```python
from build123d import *

# Parameters (mm, degrees)
BOSS_EXTRUDE1_DEPTH = 914.4
SKETCH2_R           = 1.5875
CUT_EXTRUDE2_DEPTH  = 2.794
SKETCH4_R           = 1.5875
SKETCH4_R_2         = 3.175
CUT_EXTRUDE3_DEPTH  = 8.89
SKETCH10_W          = 19.05
SKETCH10_H          = 914.4
CUT_EXTRUDE4_DEPTH  = 915.79678891
CUT_EXTRUDE5_REACH  = 916.797
SKETCH11_R          = 3.175


with BuildPart() as part:
    # Sketch1 → Boss-Extrude1 (new body)
    with BuildSketch(Plane.XY):
        Polygon((0, 0), (0, 19.05), (1.5875, 19.05), (1.5875, 1.5875), (19.05, 1.5875), (19.05, 0), align=None)
    boss_extrude1 = extrude(amount=-BOSS_EXTRUDE1_DEPTH)

    # Sketch2 → Cut-Extrude2 (cut)
    with BuildSketch(Plane(origin=(0, 1.5875, 0), x_dir=(1, 0, 0), z_dir=(0, 1, 0))):
        with Locations(Location((9.525, 9.525, 0), (0, 0, 270))):
            Circle(SKETCH2_R)
        with Locations(Location((9.525, 904.875, 0), (0, 0, 270))):
            Circle(SKETCH2_R)
    cut_extrude2 = extrude(amount=-CUT_EXTRUDE2_DEPTH, mode=Mode.SUBTRACT)

    # Sketch4 → Cut-Extrude3 (cut)
    with BuildSketch(Plane(origin=(1.5875, 0, 0), x_dir=(0, 0, -1), z_dir=(1, 0, 0))):
        with Locations((9.525, 9.525)):
            Circle(SKETCH4_R)
        with Locations((904.875, 9.525)):
            Circle(SKETCH4_R)
        with Locations((254, 9.525)):
            Circle(SKETCH4_R_2)
        with Locations((285.75, 9.525)):
            Circle(SKETCH4_R_2)
        with Locations((317.5, 9.525)):
            Circle(SKETCH4_R_2)
        with Locations((349.25, 9.525)):
            Circle(SKETCH4_R_2)
        with Locations((469.9, 9.525)):
            Circle(SKETCH4_R_2)
        with Locations((406.4, 9.525)):
            Circle(SKETCH4_R_2)
        with Locations((438.15, 9.525)):
            Circle(SKETCH4_R_2)
        with Locations((374.65, 9.525)):
            Circle(SKETCH4_R_2)
    cut_extrude3 = extrude(amount=-CUT_EXTRUDE3_DEPTH, mode=Mode.SUBTRACT)

    # Mirror1: Boss-Extrude1, Cut-Extrude2, Cut-Extrude3 across plane
    add(boss_extrude1.mirror(Plane(origin=(0, 19.05, -914.4), x_dir=(0, 0, 1), z_dir=(0, 1, 0))))
    add(cut_extrude2.mirror(Plane(origin=(0, 19.05, -914.4), x_dir=(0, 0, 1), z_dir=(0, 1, 0))), mode=Mode.SUBTRACT)
    add(cut_extrude3.mirror(Plane(origin=(0, 19.05, -914.4), x_dir=(0, 0, 1), z_dir=(0, 1, 0))), mode=Mode.SUBTRACT)

    # Sketch10 → Cut-Extrude4 (cut, through all)
    with BuildSketch(Plane(origin=(0, 19.05, 0), x_dir=(-1, 0, 0), z_dir=(0, -1, 0))):
        with Locations((-9.525, 457.2)):
            Rectangle(SKETCH10_W, SKETCH10_H)
    extrude(amount=-CUT_EXTRUDE4_DEPTH, mode=Mode.SUBTRACT)

    # Sketch11 → Cut-Extrude5 (cut, up to next)
    with BuildSketch(Plane.ZY, mode=Mode.PRIVATE) as cut_extrude5_sk1:
        with Locations((-228.6, 9.525)):
            Circle(SKETCH11_R)
    cut_extrude5_tool1 = extrude(cut_extrude5_sk1.sketch, amount=-CUT_EXTRUDE5_REACH, mode=Mode.PRIVATE) & part.part
    # Sketch11 → Cut-Extrude5 (cut, up to next)
    with BuildSketch(Plane.ZY, mode=Mode.PRIVATE) as cut_extrude5_sk2:
        with Locations((-495.3, 9.525)):
            Circle(SKETCH11_R)
    cut_extrude5_tool2 = extrude(cut_extrude5_sk2.sketch, amount=-CUT_EXTRUDE5_REACH, mode=Mode.PRIVATE) & part.part
    add(cut_extrude5_tool1.solids().sort_by_distance((0, 9.525, -228.6))[0], mode=Mode.SUBTRACT)
    add(cut_extrude5_tool2.solids().sort_by_distance((0, 9.525, -495.3))[0], mode=Mode.SUBTRACT)


solid = part.part
```
Read the model definition and answer for the solid it produces. Units are mm, in the model's axes. A direction names the side the tool comes from. Coordinates: 2 decimals unless noted, no trailing zeros. Order: outer loops, then holes, each group sorted by start corner. A loop starts at its lowest first (then second) coordinate and runs counter-clockwise, first axis right, second up. Notation, with made-up numbers: (18.5, -8.75) - (30.5, -8.75) arc R27 ccw to (30.5, 15.25) - close; hole circle Ø6 at (77, -4). An arc over 180 degrees is marked (long way). Answer as a JSON object with one key per item and string values. Group by question number.
Item 1: Section B-B (x = 15) is taken. Give the vertices of the cut face in (y, z), plus the area to 3 significant figures.
Item 2: Section A-A (z = -523.5) is taken. Give the vertices of the cut face in (x, y).
Item 3: A tool of negligible diameter and unlimited length cuts with its end or side. For faces 1 (the face through (10, 1.588, -451)), 2 (the face through (0, 10, -451)), from which of +Z, -Z, +X, -X, +Y, -Y can it reach the whole face along a straight path? Write none if from no direction.
Item 4: Consider probe 1 along Y at (x, z) = (11.5, -403.5); probe 2 along Y at (x, z) = (1.05, -469.9). Determine where each line is inside the solid, lowest interval first. Write a range as from..to.
Item 5: Flat-ended cylindrical pins translate along their axes: P1, Ø7.5, axis at y = 9.525, z = -406.4, coming from the +X side; P2, Ø8.5, axis at x = 9.5, z = -275, coming from the +Y side. Find the tip coordinate at first contact, or state that the pin passes through.
Results are:
{
 "1": {"outline": "(0, -914.4) - (1.59, -914.4) - (1.59, 0) - (0, 0) - close", "area": "1,450 mm^2"},
 "2": {"outline": "(0, 0) - (19.05, 0) - (19.05, 1.59) - (1.59, 1.59) - (1.59, 19.05) - (0, 19.05) - close"},
 "3": {"face 1": "+Z, -Z, +X, +Y", "face 2": "+Z, -Z, -X, +Y, -Y"},
 "4": {"probe 1": "y = 0..1.59", "probe 2": "y = 0..6.35, 12.7..19.05"},
 "5": {"P1": "stops at x = 1.59", "P2": "stops at y = 1.59"}
}
